Design review of the part built by this model. Coordinates are the model's own, in mm. Face numbers are marked on the shaded views. A direction names the side the tool comes from. Coordinates: 2 decimals unless noted, no trailing zeros. Order: outer loops, then holes, each group sorted by start corner. A loop starts at its lowest first (then second) coordinate and runs counter-clockwise, first axis right, second up. Notation, with made-up numbers: (73, 38) -> (119, 38) arc R24 cw to (119, 68) -> close; hole circle Ø9 at (8.5, -21.75). An arc over 180 degrees is marked (long way). Use a Markdown table: item, result. Add a question column.
Q1. Add section D-D (y = 8). State the section outline as (x, z) points.
Q2. Machinability: for the marked faces 1 and 2, which of the approach directions +Z, -Z, +X, -X, +Y, -Y give a long, thin tool a straight path to every point of the face, cutting with its end or side? Answer none if there is none.
Q3. Insertion check: pin 1 (6 mm diameter, centred on y = 3.5, z = -23.5, fed in from -X); pin 2 (2.5 mm diameter, centred on x = -1.01, z = -28.24, fed in from -Y); pin 3 (5 mm diameter, centred on x = -2.5, y = 6, fed in from -Z); pin 4 (5 mm diameter, centred on x = -2.5, z = -26, fed in from +Y). Each pin has a flat end and moves straight along its axis. Give the tip position at first contact, or say it passes through.
Q4. Wall thickness on probe 1 along Y at (x, z) = (0.5, -4.5); probe 2 along Z at (x, y) = (-1, 8); probe 3 along X at (y, z) = (0.5, -27): over which ranges is each line inside the solid? List them lowest first.
Q5. Add section C-C (z = -23). State the section outline as (x, y) points, then the cut area to 3 significant figures.
Q6. Add section A-A (y = 6). State the section outline as (x, z) points, then the cut area to 3 significant figures.
Q7. Add section B-B (x = 2). State the section outline as (y, z) points.
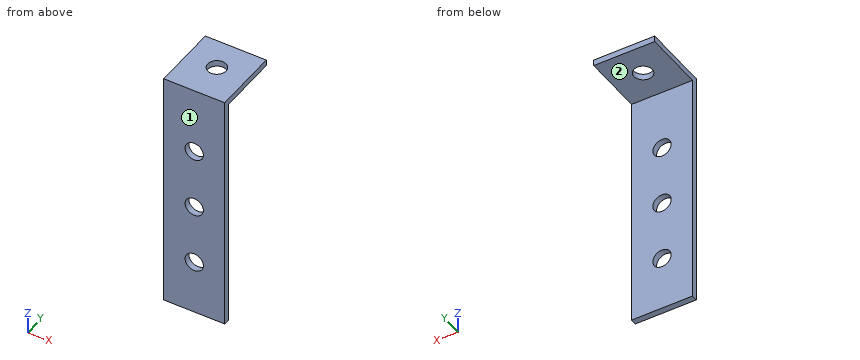
Autodesk Inventor part; units mm, degrees
ref_plane "YZ Plane" through (0, 0, 0) normal (1, 0, 0) x (0, 1, 0)
ref_plane "XZ Plane" through (0, 0, 0) normal (0, 1, 0) x (-1, 0, 0)
ref_plane "XY Plane" through (0, 0, 0) normal (0, 0, 1) x (1, 0, 0)
sketch "草图1" plane through (0, 0, 0) normal (0, 1, 0) x (-1, 0, 0)
  line L0 (6.0123, 2.7607) -> (-3.9877, 2.7607)
  line L1 (-3.9877, 2.7607) -> (-3.9877, -37.2393)
  line L2 (-3.9877, -37.2393) -> (6.0123, -37.2393)
  line L3 (6.0123, -37.2393) -> (6.0123, 2.7607)
  point P0 (0, 0)
  dimension "d0" = 40
  dimension "d1" = 10
extrude "拉伸1" add sketch "草图1" along normal blind 1
sketch "草图2" plane through (0, 1, 0) normal (0, 1, 0) x (1, 0, 0)
  line L0 (-6.0123, 37.2393) -> (-6.0123, -2.7607)
  line L1 (3.9877, -2.7607) -> (3.9877, 37.2393)
  line L2 (-6.0123, -2.7607) -> (3.9877, -2.7607)
  line L3 (3.9877, -2.7607) -> (3.9877, -1.7607)
  line L4 (3.9877, -1.7607) -> (-6.0123, -1.7607)
  line L5 (-6.0123, -1.7607) -> (-6.0123, -2.7607)
  point P0 (0, 0)
  point P1 (3.9877, -2.7607)
  dimension "d4" = 1
extrude "拉伸2" add sketch "草图2" along normal blind 10
sketch "草图3" plane through (0, 11, 0) normal (0, 1, 0) x (1, 0, 0)
  line L0 (3.9877, -1.7607) -> (-6.0123, -1.7607)
  line L1 (-1.0123, -1.7607) -> (-1.0123, 8.2393)
  circle A0 centre (-1.0123, 8.2393) radius 1.5
  line L2 (-1.0123, 8.2393) -> (-1.0123, 18.2393)
  circle A1 centre (-1.0123, 18.2393) radius 1.5
  line L3 (-1.0123, 18.2393) -> (-1.0123, 28.2393)
  circle A2 centre (-1.0123, 28.2393) radius 1.5
  point P0 (0, 0)
  dimension "d7" = 10
  dimension "d8" = 3
  dimension "d15" = 10
  dimension "d16" = 3
  dimension "d17" = 10
  dimension "d18" = 3
extrude "拉伸3" cut sketch "草图3" against normal blind 100
sketch "草图4" plane through (-6.0123, 0, 2.7607) normal (0, 0, 1) x (1, 0, 0)
  line L0 (0, 11) -> (10, 11)
  line L1 (5, 11) -> (5, 6)
  circle A0 centre (5, 6) radius 1.5
  point P0 (6.0123, 0)
  dimension "d11" = 5
  dimension "d12" = 3
extrude "拉伸4" cut sketch "草图4" against normal blind 100
equation "\"折弯半径\" = 厚度"
equation "\"折弯释压宽度\" = 厚度"
equation "\"折弯释压深度\" = 0.5 * 厚度"
equation "\"拐角释压尺寸\" = 4 * 厚度"
equation "\"最小余量\" = 2 * 厚度"
equation "\"过渡半径\" = 折弯半径"
equation "\"Jacobi半径尺寸\" = 折弯半径"
equation "\"间隙大小\" = 厚度"
Established:
| question | item | result |
|---|---|---|
| 1 | outline | (-6.01, 1.76) -> (3.99, 1.76) -> (3.99, 2.76) -> (-6.01, 2.76) -> close |
| 2 | face 1 | +Z, -Z, +X, -X, -Y |
| 2 | face 2 | -Z, +X, -X, +Y |
| 3 | pin 1 | x = -6.01 |
| 3 | pin 2 | through |
| 3 | pin 3 | z = 1.76 |
| 3 | pin 4 | y = 1 |
| 4 | probe 1 | 0 to 1 |
| 4 | probe 2 | 1.76 to 2.76 |
| 4 | probe 3 | -6.01 to -1.86, -0.17 to 3.99 |
| 5 | outline | (-6.01, 0) -> (3.99, 0) -> (3.99, 1) -> (-6.01, 1) -> close |
| 5 | area | 10.0 mm^2 |
| 6 | outline | (-6.01, 1.76) -> (-2.51, 1.76) -> (-2.51, 2.76) -> (-6.01, 2.76) -> close; (0.49, 1.76) -> (3.99, 1.76) -> (3.99, 2.76) -> (0.49, 2.76) -> close |
| 6 | area | 7.00 mm^2 |
| 7 | outline | (0, -37.24) -> (1, -37.24) -> (1, 1.76) -> (11, 1.76) -> (11, 2.76) -> (0, 2.76) -> close |
